Design review of the part built by this model. Coordinates are the model's own, in mm. Coordinates: 2 decimals unless noted, no trailing zeros. Loops run counter-clockwise (first coordinate to the right, second up) from the corner with the lowest first, then second, coordinate; pieces in that order, holes last. Notation, with made-up numbers: (-23.5, 42.25) -> (15.5, 42.25) arc R26 ccw to (15.5, 80.25) -> close; hole circle Ø11 at (-8.75, 88). An arc over 180 degrees is marked (long way). Answer in a Markdown table with one row per item.
```python
from build123d import *

# Parameters (mm, degrees)
F0_R     = 11
F1_DEPTH = 7


with BuildPart() as f1:
    # F0 (on Top) → F1 (new body)
    with BuildSketch(Plane.XY):
        with BuildLine():
            ThreePointArc((-27.08, 16.08), (-43.16, 0), (-27.08, -16.08))
            Line((-27.08, -16.08), (27.08, -16.08))
            ThreePointArc((27.08, -16.08), (43.16, 0), (27.08, 16.08))
            Line((27.08, 16.08), (-27.08, 16.08))
        make_face()
        with Locations((-27.08, 0)):
            Circle(F0_R, mode=Mode.SUBTRACT)
        with BuildLine():
            ThreePointArc((0, -11), (-11, 0), (0, 11))
            ThreePointArc((0, 11), (11, 0), (0, -11))
        make_face(mode=Mode.SUBTRACT)
        with Locations((27.08, 0)):
            Circle(F0_R, mode=Mode.SUBTRACT)
    extrude(amount=F1_DEPTH)


solid = f1.part
```
(1) Take a section at A-A on x = 0. Give the boundary of the cut face in (y, z).
Evaluation:
| item | result |
|---|---|
| outline | (-16.08, 0) -> (-11, 0) -> (-11, 7) -> (-16.08, 7) -> close; (11, 0) -> (16.08, 0) -> (16.08, 7) -> (11, 7) -> close |
(2) Take a section at C-C on y = 0. Give the boundary of the cut face in (x, z), and give its area (3 significant figures).
Evaluation:
| item | result |
|---|---|
| outline | (-43.16, 0) -> (-38.08, 0) -> (-38.08, 7) -> (-43.16, 7) -> close; (-16.08, 0) -> (-11, 0) -> (-11, 7) -> (-16.08, 7) -> close; (11, 0) -> (16.08, 0) -> (16.08, 7) -> (11, 7) -> close; (38.08, 0) -> (43.16, 0) -> (43.16, 7) -> (38.08, 7) -> close |
| area | 142 mm² |
(3) To check wall thickness, follow probe 1 along Y at (x, z) = (-27.08, 5.5); probe 2 along X at (y, z) = (3, 4.5); probe 3 along X at (y, z) = (7.5, 0.5). State the ranges of each line that lie inside material, in increasing order.
Evaluation:
| item | result |
|---|---|
| probe 1 | y = -16.08 to -11, 11 to 16.08 |
| probe 2 | x = -42.88 to -37.66, -16.5 to -10.58, 10.58 to 16.5, 37.66 to 42.88 |
| probe 3 | x = -41.3 to -35.13, -19.03 to -8.05, 8.05 to 19.03, 35.13 to 41.3 |
(4) For pin 1 (2 mm diameter, centred on y = 2, z = 5, fed in from -X); pin 2 (3 mm diameter, centred on x = -32, z = 1.5, fed in from +Y); pin 3 (1 mm diameter, centred on y = 9.5, z = 1, fed in from -X); pin 4 (13 mm diameter, centred on x = 27.08, y = 0, fed in from +Z), all flat-tipped, find the tip position at first contact; note any pin that passes through.
Evaluation:
| item | result |
|---|---|
| pin 1 | stops at x = -43.13 |
| pin 2 | stops at y = 15.71 |
| pin 3 | stops at x = -40.41 |
| pin 4 | passes through |
(5) Draft analysis for pull direction X (two halves, no side actions). For faces 1 (the flat face through (-10, 7, 7)), 2 (the cylindrical face through (43.156, -0.354, 3.451)), 3 (the cylindrical face through (-10.74, -2.38, 3.45)), 4 (the cylindrical face through (-43.156, 0.354, 3.451)), state which applies: pulls with the +X half, pulls with the -X half, needs draft (parallel to the pull), parting line crosses it, or undercut.
Evaluation:
| item | result |
|---|---|
| face 1 | needs draft |
| face 2 | pulls with the +X half |
| face 3 | undercut |
| face 4 | pulls with the -X half |
(6) Take a section at B-B on z = 4.75. Give the boundary of the cut face in (x, y), and give its area (3 significant figures).
Evaluation:
| item | result |
|---|---|
| outline | (-27.08, -16.08) -> (27.08, -16.08) arc R16.08 ccw to (27.08, 16.08) -> (-27.08, 16.08) arc R16.08 ccw to start; hole circle Ø22 at (-27.08, 0); hole circle Ø22 at (0, 0); hole circle Ø22 at (27.08, 0) |
| area | 1,410 mm² |
(7) Take a section at D-D on y = -4. Give the boundary of the cut face in (x, z).
Evaluation:
| item | result |
|---|---|
| outline | (-42.65, 0) -> (-37.33, 0) -> (-37.33, 7) -> (-42.65, 7) -> close; (-16.83, 0) -> (-10.25, 0) -> (-10.25, 7) -> (-16.83, 7) -> close; (10.25, 0) -> (16.83, 0) -> (16.83, 7) -> (10.25, 7) -> close; (37.33, 0) -> (42.65, 0) -> (42.65, 7) -> (37.33, 7) -> close |
